from build123d import *

# Parameters (mm, degrees)
SKETCH1_R           = 7
BOSS_EXTRUDE1_DEPTH = 12.5
SKETCH2_R           = 2.5
CUT_EXTRUDE1_DEPTH  = 27.888659319
SKETCH3_R           = 4
CUT_EXTRUDE2_DEPTH  = 16.945218719
CHAMFER1_SIZE       = 0.4


with BuildPart() as part:
    # Sketch1 → Boss-Extrude1 (new, symmetric)
    with BuildSketch(Plane.XY):
        Circle(SKETCH1_R)
    extrude(amount=BOSS_EXTRUDE1_DEPTH, both=True)

    # Sketch2 → Cut-Extrude1 (cut, through all)
    with BuildSketch(Plane.XY.offset(12.5)):
        Circle(SKETCH2_R)
    extrude(amount=-CUT_EXTRUDE1_DEPTH, mode=Mode.SUBTRACT)

    # Sketch3 → Cut-Extrude2 (cut, through all)
    with BuildSketch(Plane.XY):
        Circle(SKETCH3_R)
    extrude(amount=-CUT_EXTRUDE2_DEPTH, mode=Mode.SUBTRACT)

    # Chamfer1
    chamfer1_edges = [part.edges().sort_by_distance(p)[0] for p in [
        (-7, 0, -12.5),
        (-7, 0, 12.5),
    ]]
    chamfer(chamfer1_edges, length=CHAMFER1_SIZE)


solid = part.part
Can you work these out from the model? Positions are in its coordinate system, mm. A direction names the side the tool comes from. Give positions to 0.01 mm unless a question says otherwise; leave off trailing zeros. Loops run counter-clockwise (first coordinate to the right, second up) from the corner with the lowest first, then second, coordinate; pieces in that order, holes last. Notation, with made-up numbers: M -3,-35 L 37,-35 A30 cw 37,-7 Z; hole C 31,35 d7. An arc over 180 degrees is marked long. One line per item, written item: value. Start each with the question number.
1) If we section it at D-D, the plane z = -9: Write out the boundary of the cut face in (x, y), and give its area (3 significant figures).
2) On a 3-axis mill with a long thin cutter (end or side, diameter ignored), from which of +Z, -Z, +X, -X, +Y, -Y can I reach the whole of each face in a straight line? I mean faces 1 (the face through (-0.54, -2.44, 6.34)), 2 (the face through (-0.867, -3.905, -6.162)). Say none if no direction works.
3) I'm going to push flat-ended pins straight in: pin 1 (6 mm diameter, centred on x = 0, y = 0, fed in from +Z); pin 2 (2 mm diameter, centred on y = 4.5, z = 0, fed in from +X); pin 3 (3 mm diameter, centred on x = -2, z = -8.5, fed in from -Y); pin 4 (3 mm diameter, centred on y = -2.5, z = 4, fed in from -X). Where does each tip first touch, or does it pass through?
4) Thinking about a two-plate mould opening in Y: for faces 3 (the face through (3, -3, -12.5)), 4 (the face through (2, 2, 0)), 5 (the face through (6.466, -2.681, 0.169)), which applies, +Y half, -Y half, draft (parallel to the pull), parting line (faces both ways), or undercut?
5) If I drill on line 1 (Y direction, x = -1.75, z = 8.25); line 2 (X direction, y = -0.75, z = 8.5); line 3 (Y direction, x = -1.25, z = -2.5), over which ranges is the centre line in solid material (lowest first)? Write a range as [from, to].
6) If we section it at C-C, the plane z = 6: Write out the boundary of the cut face in (x, y).
7) If we section it at A-A, the plane y = 0: Write out the boundary of the cut face in (x, z).
Completed:
1. outline: C 0,0 d14; hole C 0,0 d8
1. area: 104 mm^2
2. face 1: +Z, -Z
2. face 2: -Z
3. pin 1: stops at z = 12.5
3. pin 2: stops at x = 6.06
3. pin 3: stops at y = -6.98
3. pin 4: stops at x = -6.93
4. face 3: draft
4. face 4: undercut
4. face 5: parting line
5. line 1: y = [-6.78, -1.79], [1.79, 6.78]
5. line 2: x = [-6.96, -2.38], [2.38, 6.96]
5. line 3: y = [-6.89, -3.8], [3.8, 6.89]
6. outline: C 0,0 d14; hole C 0,0 d5
7. outline: M -7,-12.1 L -6.6,-12.5 L -4,-12.5 L -4,0 L -2.5,0 L -2.5,12.5 L -6.6,12.5 L -7,12.1 Z; M 2.5,0 L 4,0 L 4,-12.5 L 6.6,-12.5 L 7,-12.1 L 7,12.1 L 6.6,12.5 L 2.5,12.5 Z
